Geometry: final body of the model. Coordinates: model frame, mm. Coordinates: 2 decimals unless noted, no trailing zeros. Write each loop counter-clockwise with the first axis right and the second up, starting at its lowest first coordinate (ties: lowest second). Pieces come first, ordered by that corner, then holes. Notation, with made-up numbers: (-13.75, 29) - (23.25, 29) arc R8 ccw to (23.25, 37) - close; hole circle Ø11 at (9.25, 48). An arc over 180 degrees is marked (long way). Put each result on its own line as item: value.
```python
from build123d import *

# Parameters (mm, degrees)
SKETCH1_W           = 3.16
SKETCH1_H           = 3.16
SKETCH1_W_2         = 2.44
SKETCH1_H_2         = 2.44
BOSS_EXTRUDE1_DEPTH = 80
SKETCH2_R           = 0.79375
CUT_EXTRUDE1_DEPTH  = 81.124722776
SKETCH3_R           = 1.5
CUT_EXTRUDE2_DEPTH  = 81.124722776


with BuildPart() as part:
    # Sketch1 → Boss-Extrude1 (new body)
    with BuildSketch(Plane(origin=(0, 0, 0), x_dir=(0, 0, -1), z_dir=(1, 0, 0))):
        with Locations((1.58, 1.58)):
            Rectangle(SKETCH1_W, SKETCH1_H)
        with Locations((1.58, 1.58)):
            Rectangle(SKETCH1_W_2, SKETCH1_H_2, mode=Mode.SUBTRACT)
    extrude(amount=BOSS_EXTRUDE1_DEPTH)

    # Sketch2 → Cut-Extrude1 (cut, through all)
    with BuildSketch(Plane.XY):
        with Locations((40, 1.16)):
            Circle(SKETCH2_R)
    extrude(amount=-CUT_EXTRUDE1_DEPTH, mode=Mode.SUBTRACT)

    # Sketch3 → Cut-Extrude2 (cut, through all)
    with BuildSketch(Plane(origin=(0, 3.16, 0), x_dir=(1, 0, 0), z_dir=(0, 1, 0))):
        with Locations(Location((10, 1.58, 0), (0, 0, 270))):
            Circle(SKETCH3_R)
    extrude(amount=-CUT_EXTRUDE2_DEPTH, mode=Mode.SUBTRACT)


solid = part.part
```
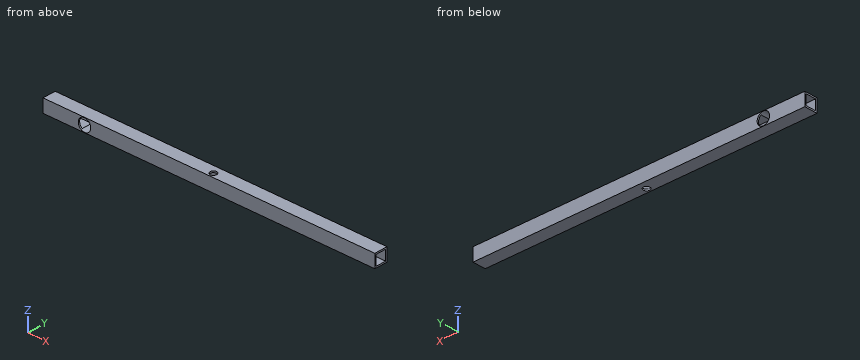
1. Ray query, probe 1 along Y at (x, z) = (26, -1.6); probe 2 along Y at (x, z) = (40, -0.3); probe 3 along Z at (x, y) = (18.5, 2.1). Return the intervals inside material, ascending. Write a range as from..to.
Answer below:
probe 1: y = 0..0.36, 2.8..3.16
probe 2: y = 0..0.37, 1.95..3.16
probe 3: z = -3.16..-2.8, -0.36..0
2. Section query D-D (x = 54.5). Return loops of the section in (y, z), then the cut area to 3 significant figures.
Answer below:
outline: (0, -3.16) - (3.16, -3.16) - (3.16, 0) - (0, 0) - close; hole (0.36, -2.8) - (2.8, -2.8) - (2.8, -0.36) - (0.36, -0.36) - close
area: 4.03 mm²
3. Section query A-A (x = 10). Return loops of the section in (y, z), then the cut area to 3 significant figures.
Answer below:
outline: (0, -3.16) - (3.16, -3.16) - (3.16, -3.08) - (0, -3.08) - close; (0, -0.08) - (3.16, -0.08) - (3.16, 0) - (0, 0) - close
area: 0.506 mm²
4. Section query C-C (z = -1.58). Return loops of the section in (x, y).
Answer below:
outline: (0, 0) - (8.5, 0) - (8.5, 0.36) - (0, 0.36) - close; (0, 2.8) - (8.5, 2.8) - (8.5, 3.16) - (0, 3.16) - close; (11.5, 0) - (80, 0) - (80, 0.36) - (11.5, 0.36) - close; (11.5, 2.8) - (80, 2.8) - (80, 3.16) - (11.5, 3.16) - close
5. Section query B-B (y = 1.16). Return loops of the section in (x, z).
Answer below:
outline: (0, -3.16) - (39.21, -3.16) - (39.21, -2.8) - (10.87, -2.8) arc R1.5 cw to (9.13, -2.8) - (0, -2.8) - close; (0, -0.36) - (9.13, -0.36) arc R1.5 cw to (10.87, -0.36) - (39.21, -0.36) - (39.21, 0) - (0, 0) - close; (40.79, -3.16) - (80, -3.16) - (80, -2.8) - (40.79, -2.8) - close; (40.79, -0.36) - (80, -0.36) - (80, 0) - (40.79, 0) - close
